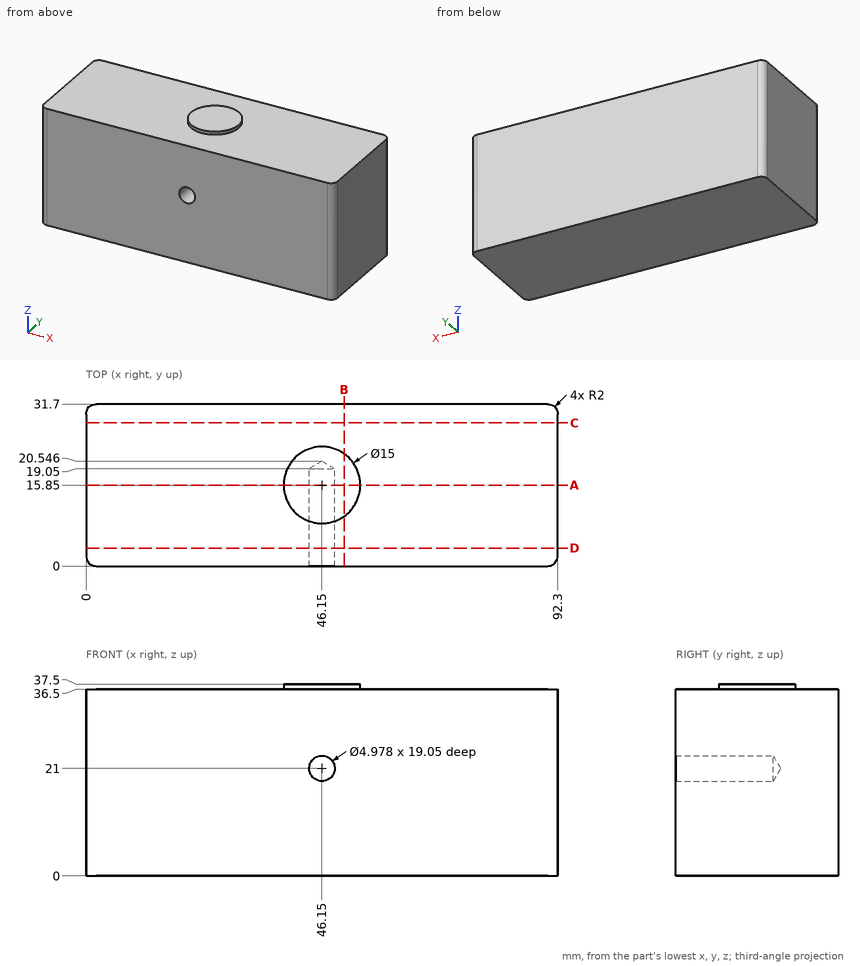
The figure shows three views and two pictorial views of one solid part (mm, origin at its lowest corner). Answer the questions. Coordinates: 2 decimals unless noted, no trailing zeros. Write each loop counter-clockwise with the first axis right and the second up, starting at its lowest first coordinate (ties: lowest second). Pieces come first, ordered by that corner, then holes.
1. The part is cut by section A-A, the plane y = 15.85. Write down the section's boundary in (x, z), and give its area (3 significant figures).
Results list:
outline: (0, 0) - (92.3, 0) - (92.3, 36.5) - (53.65, 36.5) - (53.65, 37.5) - (38.65, 37.5) - (38.65, 36.5) - (0, 36.5) - close; hole circle Ø4.98 at (46.15, 21)
area: 3,360 mm2
2. Consider line 1 along X through (y, z) = (10, 21); line 2 along Z through (x, y) = (46.15, 15); line 3 along Z through (x, y) = (46.15, 7.25). Determine where each line is inside the solid, lowest interval first.
Results list:
line 1: x = 0 to 43.66, 48.64 to 92.3
line 2: z = 0 to 18.51, 23.49 to 37.5
line 3: z = 0 to 18.51, 23.49 to 36.5
3. The part is cut by section B-B, the plane x = 50.5. Write down the section's boundary in (y, z).
Results list:
outline: (0, 0) - (31.7, 0) - (31.7, 36.5) - (21.96, 36.5) - (21.96, 37.5) - (9.74, 37.5) - (9.74, 36.5) - (0, 36.5) - close
4. Flat-ended cylindrical pins translate along their axes: pin 1 (12 mm diameter, centred on x = 57, y = 22, fed in from +Z); pin 2 (3 mm diameter, centred on x = 23, y = 9, fed in from +Z). Find the tip coordinate at first contact, or state that the pin passes through.
Results list:
pin 1: stops at z = 37.5
pin 2: stops at z = 36.5
5. The part is cut by section D-D, the plane y = 3.5. Write down the section's boundary in (x, z), and give its area (3 significant figures).
Results list:
outline: (0, 0) - (92.3, 0) - (92.3, 36.5) - (0, 36.5) - close; hole circle Ø4.98 at (46.15, 21)
area: 3,350 mm2
6. The part is cut by section C-C, the plane y = 28. Write down the section's boundary in (x, z), and give its area (3 significant figures).
Results list:
outline: (0, 0) - (92.3, 0) - (92.3, 36.5) - (0, 36.5) - close
area: 3,370 mm2
